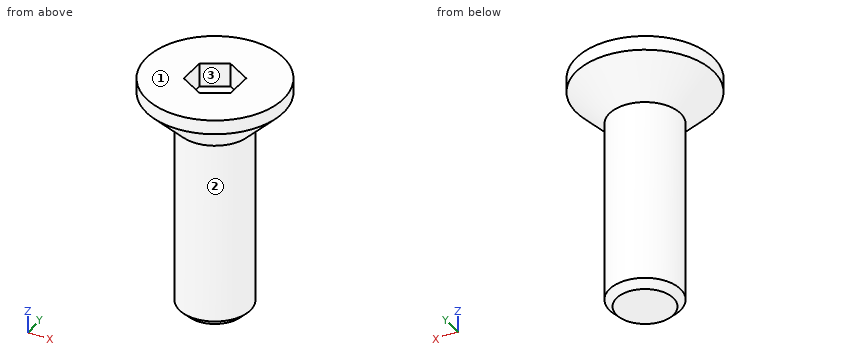
from build123d import *

# Parameters (mm, degrees)
SCHNITT_LINEAR_AUSTRAGEN1_DEPTH = 1
FASE1_SIZE                      = 0.3


with BuildPart() as part:
    # Skizze1 → Rotation1 (revolve)
    with BuildSketch(Plane(origin=(0, 0, 0), x_dir=(0, 0, -1), z_dir=(1, 0, 0))):
        Polygon((0, 0), (0, 2.9), (0.6, 2.9), (2, 1.5), (10, 1.5), (10, 0), align=None)
    revolve(axis=Axis((0, 0, 31.763581507), (0, 0, -1)))

    # Skizze3 → Schnitt-Linear austragen1 (cut)
    with BuildSketch(Plane.XY):
        Polygon((1, -0.577350269), (1, 0.577350269), (0, 1.154700538), (-1, 0.577350269), (-1, -0.577350269), (0, -1.154700538), align=None)
    extrude(amount=-SCHNITT_LINEAR_AUSTRAGEN1_DEPTH, mode=Mode.SUBTRACT)

    # Fase1
    fase1_edges = [part.edges().sort_by_distance(p)[0] for p in [
        (0, -1.5, -10),
    ]]
    chamfer(fase1_edges, length=FASE1_SIZE)


solid = part.part
Could you check a few things on this model? Use its own coordinates, in mm. Face numbers are marked on the shaded views. Round coordinates to 2 decimals unless told otherwise and drop trailing zeros. Order: outer loops, then holes, each group sorted by start corner. A loop starts at its lowest first (then second) coordinate and runs counter-clockwise, first axis right, second up.
Q1. I'm going to push flat-ended pins straight in: P1, Ø1, axis at x = -2, y = 0.5, coming from the -Z side; P2, Ø1, axis at x = -1.5, z = -6, coming from the -Y side. Where does each tip first touch, or does it pass through?
Geometry says:
P1: stops at z = -1.94
P2: stops at y = -1.12
Q2. Imagine slicing it at C-C, the plane z = -1.75. List the corners of the cut face in (x, y) for me, then the cut area to 3 significant figures.
Geometry says:
outline: circle Ø3.5 at (0, 0)
area: 9.62 mm2
Q3. Imagine slicing it at B-B, the plane z = -8.5. List the corners of the cut face in (x, y) for me.
Geometry says:
outline: circle Ø3 at (0, 0)
Q4. Thinking about a two-plate mould opening in Y: for the marked faces 1, 2 and 3, which applies, released by +Y, released by -Y, zero draft, split by the parting line, or undercut?
Geometry says:
face 1: zero draft
face 2: split by the parting line
face 3: undercut
Q5. Imagine slicing it at A-A, the plane y = 0. List the corners of the cut face in (x, z) for me.
Geometry says:
outline: (-2.9, -0.6) - (-1.5, -2) - (-1.5, -9.7) - (-1.2, -10) - (1.2, -10) - (1.5, -9.7) - (1.5, -2) - (2.9, -0.6) - (2.9, 0) - (1, 0) - (1, -1) - (-1, -1) - (-1, 0) - (-2.9, 0) - close
Q6. Please list where these lines run through material, in increasing order: probe 1 along Z at (x, y) = (0.4, 0.3); probe 2 along Y at (x, z) = (2.05, -0.75); probe 3 along Z at (x, y) = (1.75, -0.6).
Geometry says:
probe 1: z = -10 to -1
probe 2: y = -1.83 to 1.83
probe 3: z = -1.65 to 0
